Geometry check sheet. Reference: the model listing, model coordinates, mm. A direction names the side the tool comes from. Round coordinates to 2 decimals unless told otherwise and drop trailing zeros. Order: outer loops, then holes, each group sorted by start corner. A loop starts at its lowest first (then second) coordinate and runs counter-clockwise, first axis right, second up. Notation, with made-up numbers: (16, 45.25) -> (24, 45.25) arc R33 ccw to (24, 83.25) -> close; hole circle Ø2 at (1, 16.5). An arc over 180 degrees is marked (long way). Use a Markdown table: item, result. Add a question column.
Item 1: Set-up check for faces 5 (the flat face through (-19, 4, -5)), 6 (the flat face through (-19, 4, 0)): record each of +Z, -Z, +X, -X, +Y, -Y from which the full face is reachable in a straight line by a thin tool's end or side.
Item 2: Material ranges on probe 1 along Z at (x, y) = (6.05, 0); probe 2 along Z at (x, y) = (8.45, 0); probe 3 along Z at (x, y) = (-10, 1.25), recorded low to high. Write a range as [from, to].
Item 3: Sectioned sample at C-C, the plane z = 20. Record the cut outline in (x, y).
Item 4: Sectioned sample at D-D, the plane y = 3.5. Record the cut outline in (x, z), and give its area (3 significant figures).
Item 5: Mould release check, pull along Y, two halves, no side actions. Record for faces 1 (the flat face through (-4, -15, -1)), 2 (the cylindrical face through (-20, 0, -2)), 3 (the cylindrical face through (6.99, -0.21, -2.15)), 4 (the cylindrical face through (7.46, -0.33, 22.48)): pulls with the +Y half, pulls with the -Y half, needs draft (parallel to the pull), parting line crosses it, or undercut.
Item 6: Gauge pin test, flat ends, axial feed: pin 1 Ø13 at (x, y) = (-15, 0) entering from +Z; pin 2 Ø10 at (y, z) = (6.5, 11) entering from -X; pin 3 Ø1.5 at (x, y) = (0, -0.5) entering from +Z. Record the tip position at first contact, or that the pin passes through.
Item 7: Sectioned sample at A-A, the plane y = 0. Record the cut outline in (x, z), and give its area (3 significant figures).
Item 8: Sectioned sample at B-B, the plane x = -15. Record the cut outline in (y, z).
from build123d import *

# Parameters (mm, degrees)
SKETCH1_W          = 30
SKETCH1_H          = 30
BASE_FLANGE1_DEPTH = 5
SKETCH6_R          = 5
CUT_EXTRUDE1_DEPTH = 34.911649916
EDGE_FLANGE1_DEPTH = 30
HOLE1_START        = 5
HOLE1_OUTLINE_R    = 2.5
HOLE1_DEPTH        = 5
LPATTERN1_COUNT    = 2
LPATTERN1_PITCH    = 10


# Read off the part's stored shape, not the designer's step: Hole1
# Sheet-metal steps are written as plain solids
with BuildPart() as part:
    # Sketch1 → Base-Flange1 (new body)
    with BuildSketch(Plane.XY):
        with Locations((-15, 0)):
            Rectangle(SKETCH1_W, SKETCH1_H)
    extrude(amount=-BASE_FLANGE1_DEPTH)

    # Sketch6 → Cut-Extrude1 (cut, through all)
    with BuildSketch(Plane.XY):
        with Locations((-15, 0)):
            Circle(SKETCH6_R)
    extrude(amount=-CUT_EXTRUDE1_DEPTH, mode=Mode.SUBTRACT)

    # Edge-Flange1 section (across the edge) → Edge-Flange1 (add)
    with BuildSketch(Plane(origin=(5, -15, 0), x_dir=(-1, 0, 0), z_dir=(0, 1, 0))):
        with BuildLine():
            Line((-5, 5), (-5, 25))
            Line((-5, 25), (0, 25))
            Line((0, 25), (0, 5))
            ThreePointArc((0, 5), (1.464466094, 1.464466094), (5, 0))
            Line((5, 0), (5, -5))
            ThreePointArc((5, -5), (-2.071067812, -2.071067812), (-5, 5))
        make_face()
    extrude(amount=EDGE_FLANGE1_DEPTH)

    # Hole1 outline → Hole1 (cut)
    with BuildSketch(Plane.YZ.offset(HOLE1_START)):
        with Locations((0, 10)):
            Circle(HOLE1_OUTLINE_R)
    hole1 = extrude(amount=HOLE1_DEPTH, mode=Mode.SUBTRACT)

    # LPattern1: Hole1 ×2
    with Locations(*[(0, 0, i * LPATTERN1_PITCH) for i in range(1, LPATTERN1_COUNT)]):
        add(hole1, mode=Mode.SUBTRACT)


solid = part.part
Found:
| question | item | result |
|---|---|---|
| 1 | face 5 | -Z, +X, -X, +Y, -Y |
| 1 | face 6 | +Z, -X, +Y, -Y |
| 2 | probe 1 | z = [-2.96, 7.5], [12.5, 17.5], [22.5, 25] |
| 2 | probe 2 | z = [-0.35, 7.5], [12.5, 17.5], [22.5, 25] |
| 2 | probe 3 | z = [-5, 0] |
| 3 | outline | (5, -15) -> (10, -15) -> (10, -2.5) -> (5, -2.5) -> close; (5, 2.5) -> (10, 2.5) -> (10, 15) -> (5, 15) -> close |
| 4 | outline | (-30, -5) -> (-18.57, -5) -> (-18.57, 0) -> (-30, 0) -> close; (-11.43, -5) -> (0, -5) arc R10 ccw to (10, 5) -> (10, 25) -> (5, 25) -> (5, 5) arc R5 cw to (0, 0) -> (-11.43, 0) -> close |
| 4 | area | 273 mm2 |
| 5 | face 1 | pulls with the -Y half |
| 5 | face 2 | undercut |
| 5 | face 3 | needs draft |
| 5 | face 4 | undercut |
| 6 | pin 1 | stops at z = 0 |
| 6 | pin 2 | stops at x = 5 |
| 6 | pin 3 | stops at z = 0.06 |
| 7 | outline | (-30, -5) -> (-20, -5) -> (-20, 0) -> (-30, 0) -> close; (-10, -5) -> (0, -5) arc R10 ccw to (10, 5) -> (10, 7.5) -> (5, 7.5) -> (5, 5) arc R5 cw to (0, 0) -> (-10, 0) -> close; (5, 12.5) -> (10, 12.5) -> (10, 17.5) -> (5, 17.5) -> close; (5, 22.5) -> (10, 22.5) -> (10, 25) -> (5, 25) -> close |
| 7 | area | 209 mm2 |
| 8 | outline | (-15, -5) -> (-5, -5) -> (-5, 0) -> (-15, 0) -> close; (5, -5) -> (15, -5) -> (15, 0) -> (5, 0) -> close |
